```python
from build123d import *

# Parameters (mm, degrees)
F0_W     = 10
F0_H     = 8
F1_DEPTH = 5
F3_DEPTH = 10.001
F4_R     = 2.5
F5_DEPTH = 9
F6_R     = 2
F7_R     = 1.49999


# Not quite as in the source:
# - a fillet or chamfer is up to 0.001 mm smaller than in the source, because OpenCascade refuses the exact size


with BuildPart() as f1:
    # F0 (on Front) → F1 (new body, symmetric)
    with BuildSketch(Plane.XZ):
        Rectangle(F0_W, F0_H)
    extrude(amount=F1_DEPTH, both=True)

    # F2 (on face) → F3 (cut, through all)
    with BuildSketch(Plane.XZ.offset(5)):
        Polygon((3, -4), (-5, 4), (-5, -4), align=None)
    extrude(amount=-F3_DEPTH, mode=Mode.SUBTRACT)

    # F4 (on face) → F5 (join)
    with BuildSketch(Plane.YZ.offset(5)):
        Circle(F4_R)
    extrude(amount=F5_DEPTH)

    # F6
    f6_edges = [f1.edges().sort_by_distance(p)[0] for p in [
        (0, -5, 4),
        (0, 5, 4),
        (4, -5, -4),
        (4, 5, -4),
    ]]
    fillet(f6_edges, radius=F6_R)

    # F7 (radius 1.5 in the source; OpenCascade refuses exactly that, so slightly less here)
    f7_edges = [f1.edges().sort_by_distance(p)[0] for p in [
        (5, -5, 0),
    ]]
    fillet(f7_edges, radius=F7_R)


solid = f1.part
```
Design review of the part built by this model. Coordinates are the model's own, in mm. A direction names the side the tool comes from. Coordinates: 2 decimals unless noted, no trailing zeros. Order: outer loops, then holes, each group sorted by start corner. A loop starts at its lowest first (then second) coordinate and runs counter-clockwise, first axis right, second up.
1) Clearance check with flat-ended pins moving along their axes: pin 1 (1 mm diameter, centred on x = 11.5, z = -1.5, fed in from +Y); pin 2 (3 mm diameter, centred on y = 1, z = 0.5, fed in from -X); pin 3 (1 mm diameter, centred on x = 0.5, y = -3.5, fed in from -Z). State where each tip first meets the part, or that it passes through.
2) Take a section at A-A, the plane z = 1.5. Give the boundary of the cut face in (x, y).
3) Take a section at C-C, the plane x = 9.25. Give the boundary of the cut face in (y, z).
4) For faces 1 (the cylindrical face through (9.44, -0.54, -2.44)), 2 (the flat face through (1, 5, 0)), list the 3-axis set-ups (+Z, -Z, +X, -X, +Y, -Y) from which the entire face can be reached by the end or side of a thin tool; tool diameter is ignored.
5) Wall thickness on line 1 along Z through (x, y) = (8.5, 1.5); line 2 along X through (y, z) = (2.5, 1); line 3 along Z through (x, y) = (-3.5, -2.5): over which ranges is each line inside the solid? List them lowest first.
Returned:
1. pin 1: stops at y = 2.29
1. pin 2: stops at x = -3
1. pin 3: stops at z = -2
2. outline: (-2.5, -5) - (3.5, -5) arc R1.5 ccw to (5, -3.5) - (5, -2) - (14, -2) - (14, 2) - (5, 2) - (5, 3.5) arc R1.5 ccw to (3.5, 5) - (-2.5, 5) - close
3. outline: circle Ø5 at (0, 0)
4. face 1: +X
4. face 2: +Z, -Z, +X, -X, +Y
5. line 1: z = -2 to 2
5. line 2: x = -2 to 5
5. line 3: z = 2.5 to 4
